The figure shows three views and two pictorial views of one solid part (mm, origin at its lowest corner). Answer the questions. Round coordinates to 2 decimals unless told otherwise and drop trailing zeros. Order: outer loops, then holes, each group sorted by start corner. A loop starts at its lowest first (then second) coordinate and runs counter-clockwise, first axis right, second up. Notation, with made-up numbers: M 13,86.25 L 28,86.25 A11 ccw 28,106.25 Z; hole C -15.75,33.25 d11. An arc over 180 degrees is marked long. Return JSON: item names as keys, results as strings.
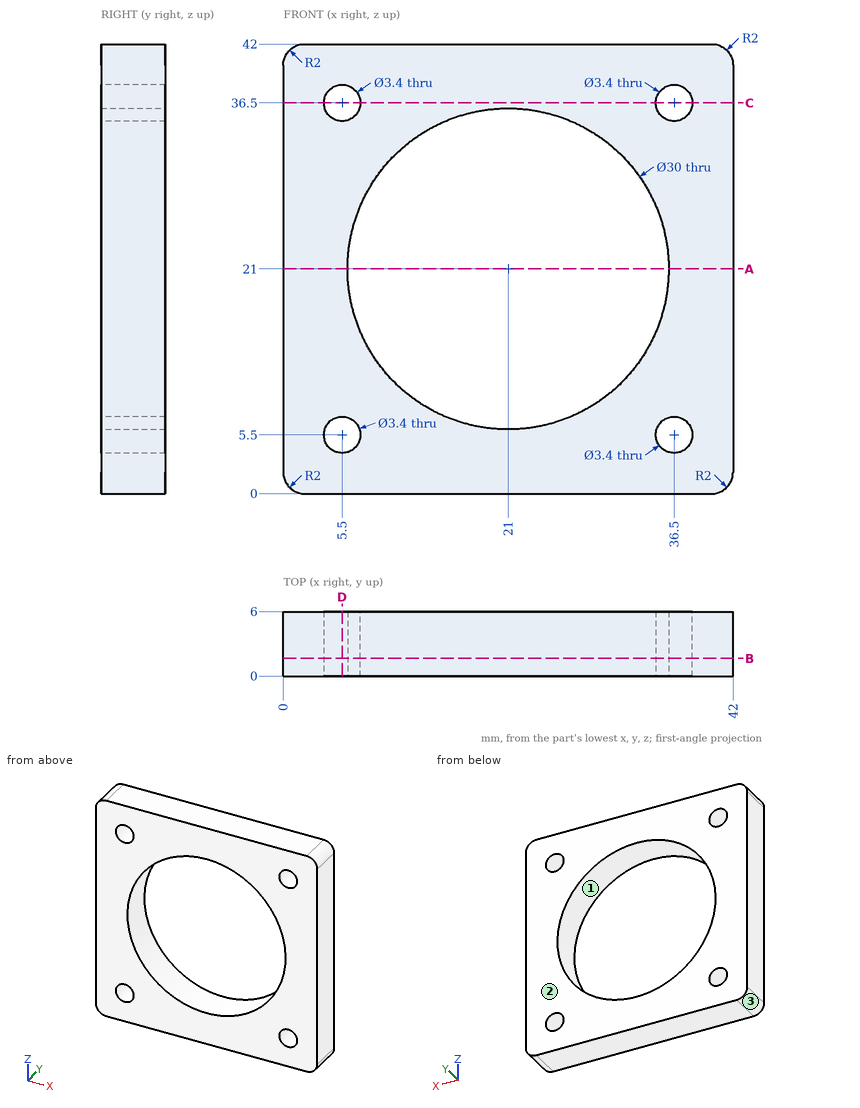
Item 1: Find section B-B (y = 1.65). Determine the outline of the cut face in (x, z), plus the area to 3 significant figures.
Output:
{"outline": "M 0,2 A2 ccw 2,0 L 40,0 A2 ccw 42,2 L 42,40 A2 ccw 40,42 L 2,42 A2 ccw 0,40 Z; hole C 5.5,5.5 d3.4; hole C 5.5,36.5 d3.4; hole C 21,21 d30; hole C 36.5,5.5 d3.4; hole C 36.5,36.5 d3.4", "area": "1,020 mm^2"}
Item 2: Find section A-A (z = 21). Determine the outline of the cut face in (x, y).
Output:
{"outline": "M 0,0 L 6,0 L 6,6 L 0,6 Z; M 36,0 L 42,0 L 42,6 L 36,6 Z"}
Item 3: Find section D-D (x = 5.5). Determine the outline of the cut face in (y, z), plus the area to 3 significant figures.
Output:
{"outline": "M 0,0 L 6,0 L 6,3.8 L 0,3.8 Z; M 0,7.2 L 6,7.2 L 6,34.8 L 0,34.8 Z; M 0,38.2 L 6,38.2 L 6,42 L 0,42 Z", "area": "211 mm^2"}
Item 4: The mould has two halves that part along X. Classify the marked faces 1, 2 and 3: pulls with the +X half, pulls with the -X half, needs draft (parallel to the pull), parting line crosses it, or undercut.
Output:
{"face 1": "undercut", "face 2": "needs draft", "face 3": "pulls with the -X half"}
Item 5: Consider line 1 along Z through (x, y) = (5.5, 1.2); line 2 along X through (y, z) = (3.65, 21). Determine where each line is inside the solid, lowest interval first. Write a range as [from, to].
Output:
{"line 1": "z = [0, 3.8], [7.2, 34.8], [38.2, 42]", "line 2": "x = [0, 6], [36, 42]"}
Item 6: Find section C-C (z = 36.5). Determine the outline of the cut face in (x, y).
Output:
{"outline": "M 0,0 L 3.8,0 L 3.8,6 L 0,6 Z; M 7.2,0 L 34.8,0 L 34.8,6 L 7.2,6 Z; M 38.2,0 L 42,0 L 42,6 L 38.2,6 Z"}
